```python
from build123d import *

# Parameters (mm, degrees)
SKETCH1_W           = 10
SKETCH1_H           = 70
SKETCH1_R           = 2.5
BOSS_EXTRUDE1_DEPTH = 5
SKETCH2_W           = 5
SKETCH2_H           = 10
BOSS_EXTRUDE2_DEPTH = 90
BOSS_EXTRUDE3_DEPTH = 4
SKETCH5_W           = 10
SKETCH5_H           = 5
BOSS_EXTRUDE4_DEPTH = 80
BOSS_EXTRUDE5_DEPTH = 10
SKETCH7_R           = 2.5
CUT_EXTRUDE1_DEPTH  = 10
BOSS_EXTRUDE6_DEPTH = 10
SKETCH9_R           = 2.5
CUT_EXTRUDE2_DEPTH  = 10
CUT_EXTRUDE3_DEPTH  = 1
FILLET1_R           = 20


with BuildPart() as part:
    # Sketch1 → Boss-Extrude1 (new body)
    with BuildSketch(Plane.XY):
        with Locations((-11.402877698, -2.158273381)):
            Rectangle(SKETCH1_W, SKETCH1_H)
        with Locations((-11.402877698, 22.841726619)):
            Circle(SKETCH1_R, mode=Mode.SUBTRACT)
        with Locations((-11.402877698, -27.158273381)):
            Circle(SKETCH1_R, mode=Mode.SUBTRACT)
    extrude(amount=BOSS_EXTRUDE1_DEPTH)

    # Sketch2 → Boss-Extrude2 (add)
    with BuildSketch(Plane.ZY.offset(16.402877698)):
        with Locations((2.5, 27.841726619)):
            Rectangle(SKETCH2_W, SKETCH2_H)
    extrude(amount=BOSS_EXTRUDE2_DEPTH)

    # Sketch3 → Boss-Extrude3 (add)
    with BuildSketch(Plane(origin=(0, 0, 0), x_dir=(-1, 0, 0), z_dir=(0, 0, -1))):
        Polygon((16.402877698, -27.158273381), (52.551297267, 22.841726619), (16.402877698, 22.841726619), align=None)
    extrude(amount=-BOSS_EXTRUDE3_DEPTH)

    # Sketch5 → Boss-Extrude4 (add)
    with BuildSketch(Plane(origin=(0, 32.841726619, 0), x_dir=(1, 0, 0), z_dir=(0, 1, 0))):
        with Locations((-11.402877698, -2.5)):
            Rectangle(SKETCH5_W, SKETCH5_H)
        with Locations((-101.402877698, -2.5)):
            Rectangle(SKETCH5_W, SKETCH5_H)
    extrude(amount=BOSS_EXTRUDE4_DEPTH)

    # Sketch6 → Boss-Extrude5 (add)
    with BuildSketch(Plane(origin=(-6.402877698, 0, 0), x_dir=(0, 0, -1), z_dir=(1, 0, 0))):
        with BuildLine():
            Line((-6.75, 130.009805512), (-6.75, 123.759805512))
            ThreePointArc((-6.75, 123.759805512), (-5.34531818, 124.685883055), (-3.75, 125.22040203))
            Line((-3.75, 125.22040203), (-3.75, 130.009805512))
            Line((-3.75, 130.009805512), (-6.75, 130.009805512))
        make_face()
        with BuildLine():
            ThreePointArc((-3.75, 125.22040203), (-5.34531818, 124.685883055), (-6.75, 123.759805512))
            ThreePointArc((-6.75, 123.759805512), (-8.918078893, 117.813007357), (-5, 112.841726619))
            Line((-5, 112.841726619), (0, 112.841726619))
            ThreePointArc((0, 112.841726619), (2.908326913, 115.236175343), (4, 118.841726619))
            ThreePointArc((4, 118.841726619), (3.410795209, 121.545890075), (1.75, 123.759805512))
            ThreePointArc((1.75, 123.759805512), (0.34531818, 124.685883055), (-1.25, 125.22040203))
            Line((-1.25, 125.22040203), (-1.25, 122.641397657))
            ThreePointArc((-1.25, 122.641397657), (0.740370349, 121.186934499), (1.5, 118.841726619))
            ThreePointArc((1.5, 118.841726619), (-4.84520788, 115.60135627), (-3.75, 122.641397657))
            Line((-3.75, 122.641397657), (-3.75, 125.22040203))
        make_face()
        with BuildLine():
            Line((-1.25, 130.009805512), (-1.25, 125.22040203))
            ThreePointArc((-1.25, 125.22040203), (0.34531818, 124.685883055), (1.75, 123.759805512))
            Line((1.75, 123.759805512), (1.75, 130.009805512))
            Line((1.75, 130.009805512), (-1.25, 130.009805512))
        make_face()
    extrude(amount=-BOSS_EXTRUDE5_DEPTH)

    # Sketch7 → Cut-Extrude1 (cut)
    with BuildSketch(Plane(origin=(0, 0, -1.75), x_dir=(-1, 0, 0), z_dir=(0, 0, -1))):
        with Locations((11.402877698, 126.736200343)):
            Circle(SKETCH7_R)
    extrude(amount=-CUT_EXTRUDE1_DEPTH, mode=Mode.SUBTRACT)

    # Sketch8 → Boss-Extrude6 (add)
    with BuildSketch(Plane.ZY.offset(106.402877698)):
        with BuildLine():
            ThreePointArc((1.25, 125.22040203), (-0.34531818, 124.685883055), (-1.75, 123.759805512))
            ThreePointArc((-1.75, 123.759805512), (-3.918078893, 117.813007357), (0, 112.841726619))
            Line((0, 112.841726619), (5, 112.841726619))
            ThreePointArc((5, 112.841726619), (7.908326913, 115.236175343), (9, 118.841726619))
            ThreePointArc((9, 118.841726619), (8.410795209, 121.545890075), (6.75, 123.759805512))
            ThreePointArc((6.75, 123.759805512), (5.34531818, 124.685883055), (3.75, 125.22040203))
            Line((3.75, 125.22040203), (3.75, 122.641397657))
            ThreePointArc((3.75, 122.641397657), (5.740370349, 121.186934499), (6.5, 118.841726619))
            ThreePointArc((6.5, 118.841726619), (0.15479212, 115.60135627), (1.25, 122.641397657))
            Line((1.25, 122.641397657), (1.25, 125.22040203))
        make_face()
        with BuildLine():
            Line((1.25, 130.009805512), (-1.75, 130.009805512))
            Line((-1.75, 130.009805512), (-1.75, 123.759805512))
            ThreePointArc((-1.75, 123.759805512), (-0.34531818, 124.685883055), (1.25, 125.22040203))
            Line((1.25, 125.22040203), (1.25, 130.009805512))
        make_face()
        with BuildLine():
            Line((3.75, 130.009805512), (3.75, 125.22040203))
            ThreePointArc((3.75, 125.22040203), (5.34531818, 124.685883055), (6.75, 123.759805512))
            Line((6.75, 123.759805512), (6.75, 130.009805512))
            Line((6.75, 130.009805512), (3.75, 130.009805512))
        make_face()
    extrude(amount=-BOSS_EXTRUDE6_DEPTH)

    # Sketch9 → Cut-Extrude2 (cut)
    with BuildSketch(Plane.XY.offset(6.75)):
        with Locations((-101.402877698, 126.921763381)):
            Circle(SKETCH9_R)
    extrude(amount=-CUT_EXTRUDE2_DEPTH, mode=Mode.SUBTRACT)

    # Sketch10 → Cut-Extrude3 (cut)
    with BuildSketch(Plane(origin=(0, 0, 0), x_dir=(-1, 0, 0), z_dir=(0, 0, -1))):
        Polygon((16.402877698, -27.158273381), (52.551297267, 22.841726619), (16.402877698, 22.841726619), align=None)
    extrude(amount=-CUT_EXTRUDE3_DEPTH, mode=Mode.SUBTRACT)

    # Fillet1
    fillet1_edges = [part.edges().sort_by_distance(p)[0] for p in [
        (-106.402877698, 22.841726619, 2.5),
        (-16.402877698, -27.158273381, 2.5),
        (-52.551297267, 22.841726619, 2.5),
        (-96.402877698, 32.841726619, 2.5),
        (-16.402877698, 32.841726619, 2.5),
    ]]
    fillet(fillet1_edges, radius=FILLET1_R)


solid = part.part
```
Geometry: final body of the model. Coordinates: model frame, mm. A direction names the side the tool comes from. Give positions to 0.01 mm unless a question says otherwise; leave off trailing zeros. Order: outer loops, then holes, each group sorted by start corner. A loop starts at its lowest first (then second) coordinate and runs counter-clockwise, first axis right, second up. Notation, with made-up numbers: (17, 17) -> (39, 17) arc R18 ccw to (39, 51) -> close; hole circle Ø8 at (15.25, 66). An arc over 180 degrees is marked (long way). Write each question's results on one line, items separated by ' | '. Start each with the question number.
1) Set-up query: faces 5 (the flat face through (-42, 32, 0)), 6 (the flat face through (-58.7, 22.842, 0.8)), 7 (the flat face through (-10, 129, 6.75)). Return all of +Z, -Z, +X, -X, +Y, -Y with unobstructed straight access to the full face (end or side cutting, diameter ignored); none if empty.
2) Section C-C (y = 17). Return loops of the section in (x, z), then the cut area to 3 significant figures.
3) Section B-B (y = 49). Return loops of the section in (x, z).
4) Section A-A (x = -31). Return loops of the section in (y, z).
5) Section D-D (x = -67.5). Return loops of the section in (y, z).
6) First-contact query: pin 1 (2 mm diameter, centred on x = -13.5, y = 126, fed in from +Z); pin 2 (3 mm diameter, centred on x = -11.4, y = -27.16, fed in from -Z); pin 3 (4 mm diameter, centred on x = -77, z = 5.5, fed in from -Y); pin 4 (6 mm diameter, centred on x = -65.5, y = 23, fed in from +Z). Flat tips, straight axial feed; report the tip coordinate or a pass-through.
7) Line query: line 1 (X direction, y = 121, z = -3); line 2 (Y direction, x = -11, z = 5.5); line 3 (Z direction, x = -99.5, y = 87). Output: solid intervals per line, ascending. Write a range as from..to.
8) Draft query along Y for faces 1 (the cylindrical face through (-13.245, -25.469, 2.465)), 2 (the cylindrical face through (-103, 125, 0)), 3 (the flat face through (-106.403, 87, 2)), 4 (the flat face through (-101, 130.01, 0)). Return one class per face: pulls with the +Y half, pulls with the -Y half, needs draft (parallel to the pull), parting line crosses it, or undercut.
Calculated:
1) face 5: -Z, +X, -X, -Y | face 6: -X, -Y | face 7: +Z, +X, -X, +Y
2) outline: (-48.65, 1) -> (-16.4, 1) -> (-16.4, 0) -> (-6.4, 0) -> (-6.4, 5) -> (-16.4, 5) -> (-16.4, 4) -> (-48.65, 4) -> close | area: 147 mm2
3) outline: (-106.4, 0) -> (-96.03, 0) -> (-96.03, 5) -> (-106.4, 5) -> close; (-16.78, 0) -> (-6.4, 0) -> (-6.4, 5) -> (-16.78, 5) -> close
4) outline: (-6.97, 1) -> (22.84, 1) -> (22.84, 0) -> (33.59, 0) -> (33.59, 5) -> (22.84, 5) -> (22.84, 4) -> (-6.97, 4) -> close
5) outline: (22.84, 0) -> (32.84, 0) -> (32.84, 5) -> (22.84, 5) -> close
6) pin 1: z = 6.75 | pin 2: through | pin 3: y = 22.84 | pin 4: z = 5
7) line 1: -106.4..-96.4, -16.4..-6.4 | line 2: 113.08..116.2, 121.49..124.27, 129.2..130.01 | line 3: 0..5
8) face 1: undercut | face 2: undercut | face 3: needs draft | face 4: pulls with the +Y half
